For this review, use the dimensioned drawing (mm, ordinates from the lowest corner) and the shaded views. A direction names the side the tool comes from. Round coordinates to 2 decimals unless told otherwise and drop trailing zeros. Write each loop counter-clockwise with the first axis right and the second up, starting at its lowest first coordinate (ties: lowest second). Pieces come first, ordered by that corner, then holes.
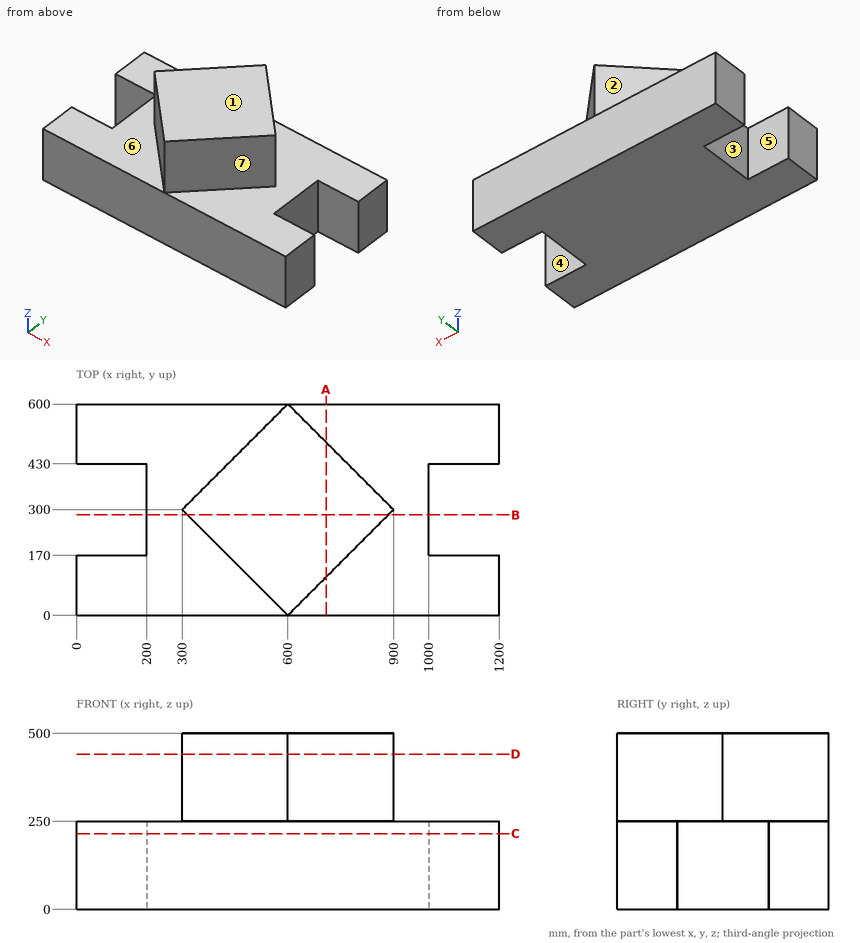
(1) For pin 1 Ø1 at (y, z) = (175, 245.5) entering from -X; pin 2 Ø2 at (x, y) = (343.5, 229.5) entering from -Z; pin 3 Ø4 at (x, z) = (457.5, 356.5) entering from +Y; pin 4 Ø4 at (x, z) = (632, 314.5) entering from +Y, all flat-tipped, find the tip position at first contact; note any pin that passes through.
Geometry check:
pin 1: stops at x = 200
pin 2: stops at z = 0
pin 3: stops at y = 459.5
pin 4: stops at y = 570
(2) We need section D-D, the plane z = 441. Give the boundary of the cut face in (x, y), and give its area (3 significant figures).
Geometry check:
outline: (300, 300) - (600, 0) - (900, 300) - (600, 600) - close
area: 180,000 mm2
(3) We need section B-B, the plane y = 285. Give the boundary of the cut face in (x, z), and give its area (4 significant figures).
Geometry check:
outline: (200, 0) - (1000, 0) - (1000, 250) - (885, 250) - (885, 500) - (315, 500) - (315, 250) - (200, 250) - close
area: 342,500 mm2
(4) For line 1 along Y through (x, z) = (57.5, 247); line 2 along Z through (x, y) = (119.5, 139); line 3 along X through (y, z) = (197.5, 80.5), list the stretches that pass through material, from the lowest coordinate up.
Geometry check:
line 1: y = 0 to 170, 430 to 600
line 2: z = 0 to 250
line 3: x = 200 to 1000
(5) We need section C-C, the plane z = 215. Give the boundary of the cut face in (x, y).
Geometry check:
outline: (0, 0) - (1200, 0) - (1200, 170) - (1000, 170) - (1000, 430) - (1200, 430) - (1200, 600) - (0, 600) - (0, 430) - (200, 430) - (200, 170) - (0, 170) - close
(6) For the marked faces 4, 5, 6 and 7, list the 3-axis set-ups (+Z, -Z, +X, -X, +Y, -Y) from which the entire face can be reached by the end or side of a thin tool; tool diameter is ignored.
Geometry check:
face 4: +Z, -Z, +X
face 5: +Z, -Z, -X
face 6: +Z, -X
face 7: +Z, +X, -Y
(7) Mouldability with a two-part tool opening along Y and no side actions: class the marked faces 1, 2 and 3 as pulls with the +Y half, pulls with the -Y half, needs draft (parallel to the pull), parting line crosses it, or undercut.
Geometry check:
face 1: needs draft
face 2: pulls with the +Y half
face 3: undercut
(8) We need section A-A, the plane x = 709. Give the boundary of the cut face in (y, z), and give its area (4 significant figures).
Geometry check:
outline: (0, 0) - (600, 0) - (600, 250) - (491, 250) - (491, 500) - (109, 500) - (109, 250) - (0, 250) - close
area: 245,500 mm2
